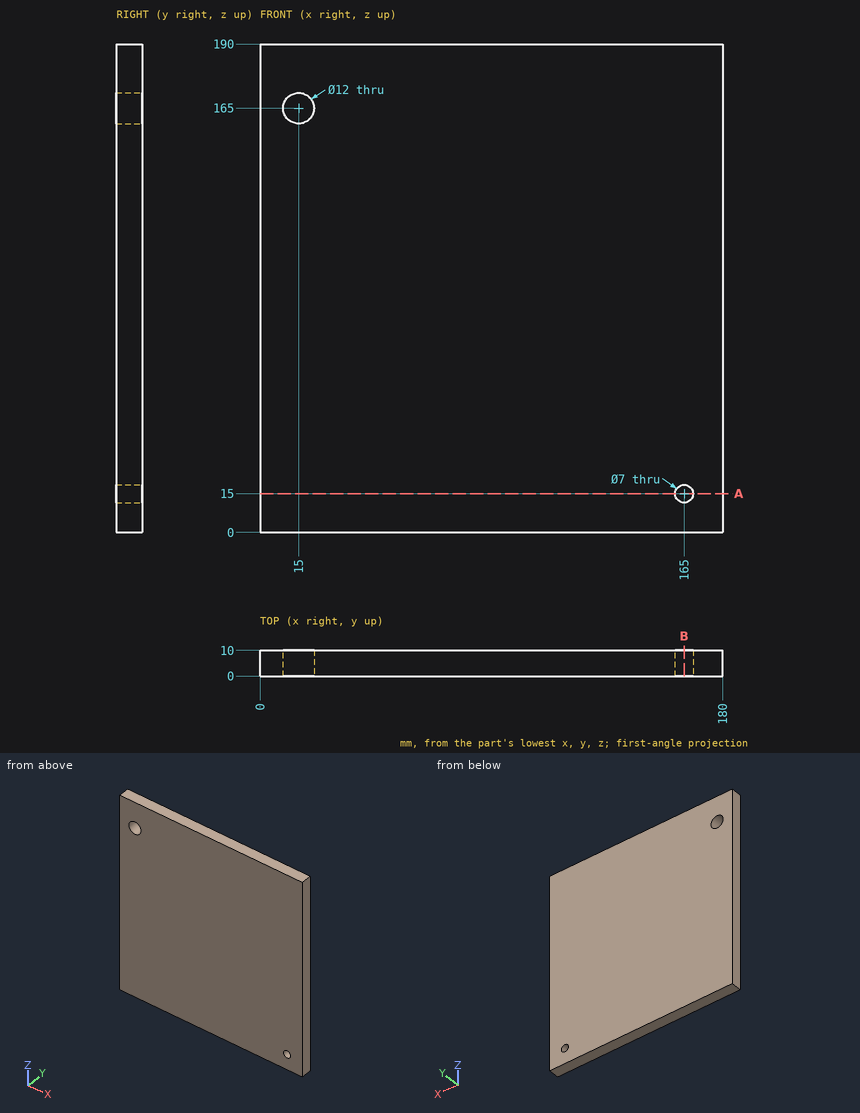
Design review of the part shown in the three views and the two pictorial views. Dimensions are in mm from the part's minimum x, y and z. Round coordinates to 2 decimals unless told otherwise and drop trailing zeros. Loops run counter-clockwise (first coordinate to the right, second up) from the corner with the lowest first, then second, coordinate; pieces in that order, holes last. Notation, with made-up numbers: (-3, 31.25) -> (17, 31.25) arc R22 cw to (17, 57.25) -> close; hole circle Ø11 at (-4.5, -23). An arc over 180 degrees is marked (long way). Use one line per item in the form item = value. Start each with the question number.
Q1. We need section B-B on x = 165. Give the boundary of the cut face in (y, z), then the cut area to 3 significant figures.
Q2. For pin 1 Ø11 at (x, z) = (15, 165) entering from -Y, flat-tipped, find the tip position at first contact; note if it passes through.
Q3. Wall thickness on line 1 along X through (y, z) = (2.5, 165); line 2 along Z through (x, y) = (15, 3); line 3 along X through (y, z) = (6, 15): over which ranges is each line inside the solid? List them lowest first. Write a range as [from, to].
Q4. We need section A-A on z = 15. Give the boundary of the cut face in (x, y).
Calculated:
q1.outline = (0, 0) -> (10, 0) -> (10, 11.5) -> (0, 11.5) -> close; (0, 18.5) -> (10, 18.5) -> (10, 190) -> (0, 190) -> close
q1.area = 1,830 mm²
q2.pin_1 = through
q3.line_1 = [0, 9], [21, 180]
q3.line_2 = [0, 159], [171, 190]
q3.line_3 = [0, 161.5], [168.5, 180]
q4.outline = (0, 0) -> (161.5, 0) -> (161.5, 10) -> (0, 10) -> close; (168.5, 0) -> (180, 0) -> (180, 10) -> (168.5, 10) -> close
